Model file for the job. Use its own axes, mm. Face numbers are marked on the shaded views. A direction names the side the tool comes from. Coordinates: 2 decimals unless noted, no trailing zeros. Order: outer loops, then holes, each group sorted by start corner. A loop starts at its lowest first (then second) coordinate and runs counter-clockwise, first axis right, second up. Notation, with made-up numbers: M -12,16 L 30,16 A21 cw 30,52 Z; hole C -39.75,-34 d7. An arc over 180 degrees is marked long. Return JSON: item names as keys, results as strings.
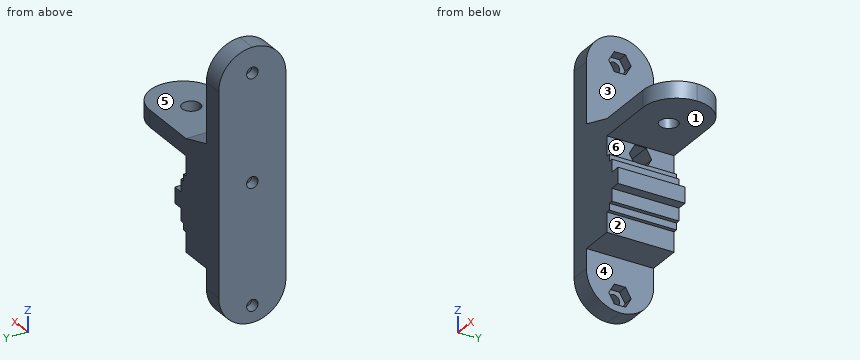
```python
from build123d import *

# Parameters (mm, degrees)
F1_DEPTH       = 20
F2_R           = 2.7
F3_DEPTH       = 5
F4_R           = 1.7
F5_DEPTH       = 16.001
F6_R           = 1.7
F7_R           = 1.7
F9_DEPTH       = 3
F8_R           = 1.7
F10_DEPTH      = 5.4
F10_DEPTH_BACK = 13
F11_R          = 9.99999


# Not quite as in the source:
# - a fillet or chamfer is up to 0.001 mm smaller than in the source, because OpenCascade refuses the exact size


with BuildPart() as f1:
    # F0 (on Front) → F1 (new body)
    with BuildSketch(Plane.XZ):
        Polygon((16, 8.8), (6, 12), (6, 40), (0, 40), (0, -40), (6, -40), (6, -24.2), (16, -24.2), (16, -18.3), (17.15, -18.3), (17.15, -16.3), (18.4, -16.3), (18.4, -12.55), (21.4, -12.55), (21.4, -7.85), (18.4, -7.85), (18.4, -4.1), (17.15, -4.1), (17.15, -2.1), (16, -2.1), (16, 3.8), (43.6, 3.8), (43.6, 8.8), align=None)
    extrude(amount=F1_DEPTH)

    # F2 (on face) → F3 (cut, through all)
    with BuildSketch(Plane(origin=(0, 0, 3.8), x_dir=(1, 0, 0), z_dir=(0, 0, -1))):
        with Locations((29.8, 10)):
            Circle(F2_R)
    extrude(amount=-F3_DEPTH, mode=Mode.SUBTRACT)

    # F4 (on face) → F5 (cut, through all)
    with BuildSketch(Plane(origin=(0, 0, 0), x_dir=(0, -1, 0), z_dir=(-1, 0, 0))):
        with Locations((10, 32.5)):
            Circle(F4_R)
        with Locations((10, 0.7)):
            Circle(F4_R)
        with Locations((10, -35)):
            Circle(F4_R)
    extrude(amount=-F5_DEPTH, mode=Mode.SUBTRACT)

    # F6 (on face) + F7 (on face) → F9 (cut)
    with BuildSketch(Plane.YZ.offset(6)):
        Polygon((-13.3486315613, 32.5), (-11.6743157806, 29.6), (-8.3256842194, 29.6), (-6.6513684387, 32.5), (-8.3256842194, 35.4), (-11.6743157806, 35.4), align=None)
        with Locations((-10, 32.5)):
            Circle(F6_R, mode=Mode.SUBTRACT)
        with Locations((-10, 32.5)):
            Circle(F6_R)
    with BuildSketch(Plane.YZ.offset(6)):
        Polygon((-8.3256842194, -37.8999999998), (-6.6513684387, -34.9999999998), (-8.3256842194, -32.0999999998), (-11.6743157806, -32.0999999998), (-13.3486315613, -34.9999999998), (-11.6743157806, -37.8999999998), align=None)
        with Locations((-10, -35)):
            Circle(F7_R, mode=Mode.SUBTRACT)
    extrude(amount=-F9_DEPTH, mode=Mode.SUBTRACT)

    # F8 (on face) → F10 (cut, two sides)
    with BuildSketch(Plane.YZ.offset(16)) as f10_sk:
        Polygon((-13.3486315613, 0.7), (-11.7320508076, -2.1), (-8.2679491924, -2.1), (-6.6513684387, 0.7), (-8.3256842194, 3.6), (-11.6743157806, 3.6), align=None)
        with Locations((-10, 0.7)):
            Circle(F8_R, mode=Mode.SUBTRACT)
        Polygon((-11.7320508076, -2.1), (-11.6743157806, -2.2), (-8.3256842194, -2.2), (-8.2679491924, -2.1), align=None)
    extrude(amount=F10_DEPTH, mode=Mode.SUBTRACT)
    extrude(f10_sk.sketch, amount=-F10_DEPTH_BACK, mode=Mode.SUBTRACT)

    # F11 (radius 10 in the source; OpenCascade refuses exactly that, so slightly less here)
    f11_edges = [f1.edges().sort_by_distance(p)[0] for p in [
        (3, -20, 40),
        (3, 0, 40),
        (3, -20, -40),
        (3, 0, -40),
        (43.6, 0, 6.3),
        (43.6, -20, 6.3),
    ]]
    fillet(f11_edges, radius=F11_R)


solid = f1.part
```
Item 1: Drop flat-ended pins along their axis: pin 1 Ø1.8 at (y, z) = (-6, -22) entering from +X; pin 2 Ø3.5 at (x, y) = (8.5, -10.5) entering from +Z; pin 3 Ø2 at (y, z) = (-4.5, 29) entering from +X. Give the stop position or say it passes through.
Check result:
{"pin 1": "stops at x = 16", "pin 2": "stops at z = 11.76", "pin 3": "stops at x = 6"}
Item 2: Saw through at A-A (x = 20.5). Write the cut outline in (y, z).
Check result:
{"outline": "M -20,-12.55 L 0,-12.55 L 0,-7.85 L -20,-7.85 Z; M -20,3.8 L 0,3.8 L 0,8.8 L -20,8.8 Z"}
Item 3: Pull direction Z, two halves, no side cores. Call the marked faces 4, 5 and 6: +Z half, -Z half, draft (parallel to the pull), parting line (faces both ways), or undercut.
Check result:
{"face 4": "draft", "face 5": "+Z half", "face 6": "undercut"}
Item 4: Saw through at D-D (x = 29.8). Write the cut outline in (y, z), and give its area (3 significant figures).
Check result:
{"outline": "M -20,3.8 L -12.7,3.8 L -12.7,8.8 L -20,8.8 Z; M -7.3,3.8 L 0,3.8 L 0,8.8 L -7.3,8.8 Z", "area": "73.0 mm2"}
Item 5: 3-axis set-ups, long thin cutter, end or side, ignore diameter. For the marked faces 1, 2 and 3: which of +Z, -Z, +X, -X, +Y, -Y reach the whole face in a straight line?
Check result:
{"face 1": "+X, +Y, -Y", "face 2": "-Z, +X, +Y, -Y", "face 3": "+Z, +X, +Y, -Y"}
Item 6: Wall check: line 1 (Z direction, x = 2, y = -10); line 2 (Y direction, x = 1.4, z = 0.7); line 3 (X direction, y = -10, z = -6.5). Give the ranges that are in metal, low to high.
Check result:
{"line 1": "z = -40 to -36.7, -33.3 to -1, 2.4 to 30.8, 34.2 to 40", "line 2": "y = -20 to -11.7, -8.3 to 0", "line 3": "x = 0 to 18.4"}
Item 7: Saw through at B-B (x = 9.5). Write the cut outline in (y, z), and give its area (3 significant figures).
Check result:
{"outline": "M -20,-24.2 L 0,-24.2 L 0,10.88 L -20,10.88 Z; hole M -13.35,0.7 L -11.67,-2.2 L -8.33,-2.2 L -6.65,0.7 L -8.33,3.6 L -11.67,3.6 Z", "area": "672 mm2"}
Item 8: Saw through at C-C (y = -18). Write the cut outline in (x, z).
Check result:
{"outline": "M 0,-36 L 6,-36 L 6,-24.2 L 16,-24.2 L 16,-18.3 L 17.15,-18.3 L 17.15,-16.3 L 18.4,-16.3 L 18.4,-12.55 L 21.4,-12.55 L 21.4,-7.85 L 18.4,-7.85 L 18.4,-4.1 L 17.15,-4.1 L 17.15,-2.1 L 16,-2.1 L 16,3.8 L 39.6,3.8 L 39.6,8.8 L 16,8.8 L 6,12 L 6,36 L 0,36 Z"}
